from build123d import *

# Parameters (mm, degrees)
SKETCH_1_R          = 1
EXTRUDE_1_DEPTH     = 1.6
EXTRUDE_START       = 1.6
SKETCH_2_W          = 26.92
SKETCH_2_H          = 9.2
EXTRUDE_2_DEPTH     = 15.2
CUT_EXTRUDE_START   = 16.8
SKETCH_3_W          = 22.86
SKETCH_3_H          = 1.6
CUT_EXTRUDE_1_DEPTH = 9
CUT_EXTRUDE_START_2 = -45
SKETCH_4_W          = 26.92
SKETCH_4_H          = 1
CUT_EXTRUDE_2_DEPTH = 0.1
CUT_EXTRUDE_START_3 = 1.6
CUT_EXTRUDE_3_DEPTH = 15.2


with BuildPart() as part:
    # 草图1 → 凸台-拉伸1 (new body)
    with BuildSketch(Plane(origin=(0, 0, 0), x_dir=(1, 0, 0), z_dir=(0, 1, 0))):
        with BuildLine():
            Line((-23, 45), (23, 45))
            ThreePointArc((23, 45), (24.414213562, 44.414213562), (25, 43))
            Line((25, 43), (25, -43))
            ThreePointArc((25, -43), (24.414213562, -44.414213562), (23, -45))
            Line((23, -45), (-23, -45))
            ThreePointArc((-23, -45), (-24.414213562, -44.414213562), (-25, -43))
            Line((-25, -43), (-25, 43))
            ThreePointArc((-25, 43), (-24.414213562, 44.414213562), (-23, 45))
        make_face()
        with Locations(Location((-23, 43, 0), (0, 0, 270))):
            Circle(SKETCH_1_R, mode=Mode.SUBTRACT)
        with Locations(Location((23, 43, 0), (0, 0, 270))):
            Circle(SKETCH_1_R, mode=Mode.SUBTRACT)
        with Locations(Location((-23, -43, 0), (0, 0, 270))):
            Circle(SKETCH_1_R, mode=Mode.SUBTRACT)
        with Locations(Location((23, -43, 0), (0, 0, 270))):
            Circle(SKETCH_1_R, mode=Mode.SUBTRACT)
    extrude(amount=EXTRUDE_1_DEPTH)

    # 草图2 → 凸台-拉伸2 (add)
    with BuildSketch(Plane(origin=(0, 0, 0), x_dir=(1, 0, 0), z_dir=(0, 1, 0)).offset(EXTRUDE_START)):
        with Locations((0, 40.4)):
            Rectangle(SKETCH_2_W, SKETCH_2_H)
    extrude(amount=EXTRUDE_2_DEPTH)

    # 草图3 → 切除-拉伸1 (cut)
    with BuildSketch(Plane(origin=(0, 0, 0), x_dir=(1, 0, 0), z_dir=(0, 1, 0)).offset(CUT_EXTRUDE_START)):
        with Locations((0, 40.4)):
            Rectangle(SKETCH_3_W, SKETCH_3_H)
    extrude(amount=-CUT_EXTRUDE_1_DEPTH, mode=Mode.SUBTRACT)

    # 草图4 → 切除-拉伸2 (cut)
    with BuildSketch(Plane.XY.offset(CUT_EXTRUDE_START_2)):
        with Locations((0, 2.1)):
            Rectangle(SKETCH_4_W, SKETCH_4_H)
    extrude(amount=CUT_EXTRUDE_2_DEPTH, mode=Mode.SUBTRACT)

    # 草图5 → 切除-拉伸3 (cut)
    with BuildSketch(Plane(origin=(0, 0, 0), x_dir=(1, 0, 0), z_dir=(0, 1, 0)).offset(CUT_EXTRUDE_START_3)):
        Polygon((13.46, 35.8), (13.46, 36.8), (12.46, 35.8), align=None)
        Polygon((13.46, 45), (13.46, 44), (12.46, 45), align=None)
        Polygon((-13.46, 45), (-13.46, 44), (-12.46, 45), align=None)
        Polygon((-13.46, 35.8), (-12.46, 35.8), (-13.46, 36.8), align=None)
    extrude(amount=CUT_EXTRUDE_3_DEPTH, mode=Mode.SUBTRACT)


solid = part.part
The listing builds one solid part. Answer for the finished solid, in the listing's coordinates (mm). A direction names the side the tool comes from. Coordinates: 2 decimals unless noted, no trailing zeros. Write each loop counter-clockwise with the first axis right and the second up, starting at its lowest first coordinate (ties: lowest second). Pieces come first, ordered by that corner, then holes. Notation, with made-up numbers: (70, 2) - (128, 2) arc R33 cw to (128, 37) - close; hole circle Ø1 at (10.25, 79.25). An arc over 180 degrees is marked (long way). Put each result on its own line as item: value.
1. The part is cut by section B-B on x = 9.5. Give the vertices of the cut face in (y, z), plus the area to 3 significant figures.
Answer sheet:
outline: (0, -45) - (1.6, -45) - (1.6, -44.9) - (2.6, -44.9) - (2.6, -45) - (16.8, -45) - (16.8, -41.2) - (7.8, -41.2) - (7.8, -39.6) - (16.8, -39.6) - (16.8, -35.8) - (1.6, -35.8) - (1.6, 45) - (0, 45) - close
area: 269 mm^2
2. Find the intervals of material crossed by line 1 along X through (y, z) = (0.5, 43); line 2 along Y through (x, z) = (18.5, -38.5); line 3 along Z through (x, y) = (9.5, 2), in increasing order. Write a range as from..to.
Answer sheet:
line 1: x = -25..-24, -22..22, 24..25
line 2: y = 0..1.6
line 3: z = -44.9..-35.8
3. A tool of negligible diameter and unlimited length cuts with its end or side. For faces 5 (the face through (13.46, 9, -40)), 6 (the face through (0, 9, -35.8)), 7 (the face through (0, 12, -39.6)), from which of +Z, -Z, +X, -X, +Y, -Y can it reach the whole face along a straight path? Write none if from no direction.
Answer sheet:
face 5: +Z, -Z, +X, +Y
face 6: +Z, +X, -X, +Y
face 7: +Y
4. The part is cut by section A-A on y = 9.75. Give the vertices of the cut face in (x, z).
Answer sheet:
outline: (-13.46, -44) - (-12.46, -45) - (12.46, -45) - (13.46, -44) - (13.46, -36.8) - (12.46, -35.8) - (-12.46, -35.8) - (-13.46, -36.8) - close; hole (-11.43, -41.2) - (11.43, -41.2) - (11.43, -39.6) - (-11.43, -39.6) - close
5. Flat-ended cylindrical pins translate along their axes: pin 1 Ø1.8 at (y, z) = (13, -40.5) entering from +X; pin 2 Ø3 at (x, z) = (-23, -43) entering from +Y; pin 3 Ø0.8 at (x, z) = (-4, -40.5) entering from +Y. Find the tip coordinate at first contact, or state that the pin passes through.
Answer sheet:
pin 1: stops at x = 13.46
pin 2: stops at y = 1.6
pin 3: stops at y = 7.8
6. The part is cut by section C-C on y = 4.25. Give the vertices of the cut face in (x, z), plus the area to 3 significant figures.
Answer sheet:
outline: (-13.46, -44) - (-12.46, -45) - (12.46, -45) - (13.46, -44) - (13.46, -36.8) - (12.46, -35.8) - (-12.46, -35.8) - (-13.46, -36.8) - close
area: 246 mm^2
7. The part is cut by section D-D on z = 33.5. Give the vertices of the cut face in (x, y).
Answer sheet:
outline: (-25, 0) - (25, 0) - (25, 1.6) - (-25, 1.6) - close
8. Determine the mould class of faces 1 (the face through (-24.4, 0.79, 44.43)), 2 (the face through (-13.46, 9, -40)), 3 (the face through (-23, 1, -42)), 4 (the face through (0, 7.8, -40)) for opening direction Z: pulls with the +Z half, pulls with the -Z half, needs draft (parallel to the pull), parting line crosses it, or undercut.
Answer sheet:
face 1: pulls with the +Z half
face 2: needs draft
face 3: undercut
face 4: undercut
